Geometry check sheet. Reference: the model listing, model coordinates, mm. A direction names the side the tool comes from. Give positions to 0.01 mm unless a question says otherwise; leave off trailing zeros. Loops run counter-clockwise (first coordinate to the right, second up) from the corner with the lowest first, then second, coordinate; pieces in that order, holes last. Notation, with made-up numbers: (40, -23.75) -> (55, -23.75) arc R29 cw to (55, 8.25) -> close; hole circle Ø6 at (36.5, 35.25). An arc over 180 degrees is marked (long way). One line per question, with ' | ' between items.
from build123d import *

# Parameters (mm, degrees)
F0_W     = 6.35
F0_H     = 38.1
F1_DEPTH = 31.75
F2_R     = 6.35
F3_DEPTH = 127
F5_DEPTH = 127
F7_DEPTH = 31.75
F8_DEPTH = 31.75


with BuildPart() as f1:
    # F0 (on Front) → F1 (new body)
    with BuildSketch(Plane.XZ):
        with Locations((-3.175, -19.05)):
            Rectangle(F0_W, F0_H)
        Polygon((-6.35, 0), (0, 0), (0, 6.35), (-76.2, 6.35), (-76.2, 0), (-69.85, 0), align=None)
        with Locations((-73.025, -19.05)):
            Rectangle(F0_W, F0_H)
    extrude(amount=F1_DEPTH)

    # F2 (on face) → F3 (cut)
    with BuildSketch(Plane.YZ):
        with Locations((-15.875, -19.05)):
            Circle(F2_R)
    extrude(amount=-F3_DEPTH, mode=Mode.SUBTRACT)

    # F4 (on face) → F5 (cut)
    with BuildSketch(Plane.YZ):
        with BuildLine():
            ThreePointArc((-15.875, -38.1), (-27.10032, -33.45032), (-31.75, -22.225))
            Line((-31.75, -22.225), (-31.75, -38.1))
            Line((-31.75, -38.1), (-15.875, -38.1))
        make_face()
        with BuildLine():
            Line((0, -38.1), (0, -22.225))
            ThreePointArc((0, -22.225), (-4.64968, -33.45032), (-15.875, -38.1))
            Line((-15.875, -38.1), (0, -38.1))
        make_face()
    extrude(amount=-F5_DEPTH, mode=Mode.SUBTRACT)

    # F6 (on face) → F7 (join)
    with BuildSketch(Plane.XZ.offset(31.75)):
        with BuildLine():
            Line((-63.5, 0), (-69.85, 0))
            Line((-69.85, 0), (-69.85, -6.35))
            ThreePointArc((-69.85, -6.35), (-67.990128, -1.859872), (-63.5, 0))
        make_face()
        with BuildLine():
            Line((-6.35, -6.35), (-6.35, 0))
            Line((-6.35, 0), (-12.7, 0))
            ThreePointArc((-12.7, 0), (-8.209872, -1.859872), (-6.35, -6.35))
        make_face()
    extrude(amount=-F7_DEPTH)

    # F6 (on face) → F8 (cut)
    with BuildSketch(Plane.XZ.offset(31.75)):
        with BuildLine():
            ThreePointArc((-76.2, 0), (-74.340128, 4.490128), (-69.85, 6.35))
            Line((-69.85, 6.35), (-76.2, 6.35))
            Line((-76.2, 6.35), (-76.2, 0))
        make_face()
        with BuildLine():
            Line((0, 6.35), (-6.35, 6.35))
            ThreePointArc((-6.35, 6.35), (-1.859872, 4.490128), (0, 0))
            Line((0, 0), (0, 6.35))
        make_face()
        with BuildLine():
            Line((-63.5, 0), (-69.85, 0))
            Line((-69.85, 0), (-69.85, -6.35))
            ThreePointArc((-69.85, -6.35), (-67.990128, -1.859872), (-63.5, 0))
        make_face()
        with BuildLine():
            Line((-6.35, -6.35), (-6.35, 0))
            Line((-6.35, 0), (-12.7, 0))
            ThreePointArc((-12.7, 0), (-8.209872, -1.859872), (-6.35, -6.35))
        make_face()
    extrude(amount=-F8_DEPTH, mode=Mode.SUBTRACT)


solid = f1.part
Item 1: Sectioned sample at D-D (y = -2.5). Record the cut outline in (x, z), plus the area to 3 significant figures.
Result:
outline: (-76.2, -30.78) -> (-69.85, -30.78) -> (-69.85, 0) -> (-6.35, 0) -> (-6.35, -30.78) -> (0, -30.78) -> (0, 0) arc R6.35 ccw to (-6.35, 6.35) -> (-69.85, 6.35) arc R6.35 ccw to (-76.2, 0) -> close | area: 857 mm2
Item 2: Sectioned sample at A-A (z = -19.05). Record the cut outline in (x, y) (3 decimals), plus the area to 3 significant figures.
Result:
outline: (-76.2, -31.75) -> (-69.85, -31.75) -> (-69.85, -22.225) -> (-76.2, -22.225) -> close; (-76.2, -9.525) -> (-69.85, -9.525) -> (-69.85, 0) -> (-76.2, 0) -> close; (-6.35, -31.75) -> (0, -31.75) -> (0, -22.225) -> (-6.35, -22.225) -> close; (-6.35, -9.525) -> (0, -9.525) -> (0, 0) -> (-6.35, 0) -> close | area: 242 mm2
Item 3: Depth check by flat-ended pin: pin 1 Ø3 at (x, y) = (-31, -13) entering from -Z. Enter the tip coordinate at first touch or a pass-through.
Result:
pin 1: z = 0
Item 4: Sectioned sample at C-C (y = -18.5). Record the cut outline in (x, z).
Result:
outline: (-76.2, -37.88) -> (-69.85, -37.88) -> (-69.85, -24.83) -> (-76.2, -24.83) -> close; (-76.2, -13.27) -> (-69.85, -13.27) -> (-69.85, 0) -> (-6.35, 0) -> (-6.35, -13.27) -> (0, -13.27) -> (0, 0) arc R6.35 ccw to (-6.35, 6.35) -> (-69.85, 6.35) arc R6.35 ccw to (-76.2, 0) -> close; (-6.35, -37.88) -> (0, -37.88) -> (0, -24.83) -> (-6.35, -24.83) -> close
Item 5: Scan lines: probe 1 along X at (y, z) = (-10, -11.5); probe 2 along Y at (x, z) = (-4, -19). Record each from-to range of solid material in increasing order.
Result:
probe 1: -76.2 to -69.85, -6.35 to 0 | probe 2: -31.75 to -22.22, -9.53 to 0
Item 6: Release check for a two-part mould opening along Y. For faces 1 (the face through (-39, 0, 2)), 2 (the face through (-3.13, -17.25, -25.25)), 3 (the face through (-6.35, -16, -11)) record: pulls with the +Y half, pulls with the -Y half, needs draft (parallel to the pull), parting line crosses it, or undercut.
Result:
face 1: pulls with the +Y half | face 2: undercut | face 3: needs draft
Item 7: Set-up check for faces 4 (the face through (-38, -16, 0)), 5 (the face through (-72.98, -17.25, -25.25)): record each of +Z, -Z, +X, -X, +Y, -Y from which the full face is reachable in a straight line by a thin tool's end or side.
Result:
face 4: -Z, +Y, -Y | face 5: +X, -X
Item 8: Sectioned sample at B-B (z = -10). Record the cut outline in (x, y).
Result:
outline: (-76.2, -31.75) -> (-69.85, -31.75) -> (-69.85, 0) -> (-76.2, 0) -> close; (-6.35, -31.75) -> (0, -31.75) -> (0, 0) -> (-6.35, 0) -> close
